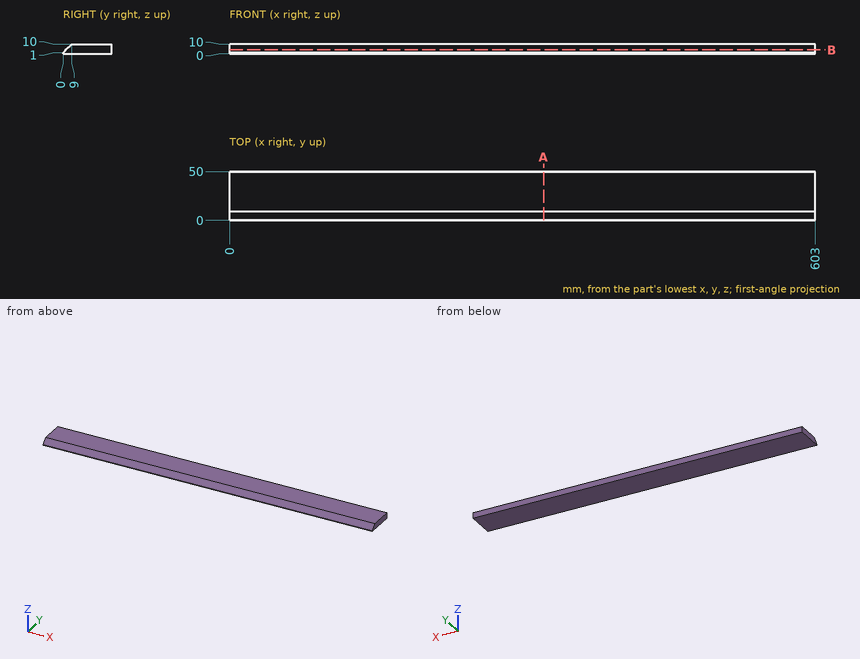
Geometry check sheet. Reference: drawing and pictorial views, mm from the part's lowest x, y, z. Give positions to 0.01 mm unless a question says otherwise; leave off trailing zeros. Loops run counter-clockwise (first coordinate to the right, second up) from the corner with the lowest first, then second, coordinate; pieces in that order, holes last. Notation, with made-up numbers: (-26, 40.25) -> (-2, 40.25) arc R27 ccw to (-2, 79.25) -> close; hole circle Ø1 at (-5, 34). An arc over 180 degrees is marked (long way). Answer in a Markdown table with one row per item. Add a question column.
1) Gauge pin test, flat end, axial feed: P1, Ø1.5, axis at x = 415.5, z = 2.5, coming from the -Y side. Record the tip position at first contact, or that the pin passes through.
2) Cross-section at A-A on x = 323.5. Record the boundary of the cut face in (y, z).
3) Cross-section at B-B on z = 4. Record the boundary of the cut face in (x, y).
4) Material ranges on probe 1 along Y at (x, z) = (272, 9); probe 2 along Y at (x, z) = (492, 8.25); probe 3 along Z at (x, y) = (552, 4.5), recorded low to high. Write a range as from..to.
Outcome:
| question | item | result |
|---|---|---|
| 1 | P1 | stops at y = 0.75 |
| 2 | outline | (0, 0) -> (50, 0) -> (50, 10) -> (9, 10) -> (0, 1) -> close |
| 3 | outline | (0, 3) -> (603, 3) -> (603, 50) -> (0, 50) -> close |
| 4 | probe 1 | y = 8..50 |
| 4 | probe 2 | y = 7.25..50 |
| 4 | probe 3 | z = 0..5.5 |
